Read the model definition and answer for the solid it produces. Units are mm, in the model's axes. Face numbers are marked on the shaded views. Give positions to 0.01 mm unless a question says otherwise; leave off trailing zeros. Order: outer loops, then holes, each group sorted by start corner. A loop starts at its lowest first (then second) coordinate and runs counter-clockwise, first axis right, second up.
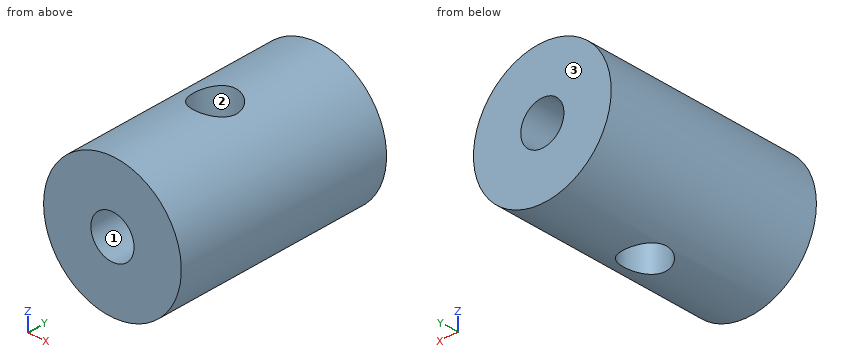
Autodesk Inventor part; units mm, degrees
ref_plane "Work Plane1" through (0, 0, 7.9375) normal (0, 0, 1) x (1, 0, 0)
ref_plane "YZ Plane" through (0, 0, 0) normal (1, 0, 0) x (0, 1, 0)
ref_plane "XZ Plane" through (0, 0, 0) normal (0, 1, 0) x (-1, 0, 0)
sketch "Sketch1" plane through (0, 0, 0) normal (0, 1, 0) x (-1, 0, 0)
  circle A0 centre (0, 0) radius 7.9375
  dimension "d0" = 15.875
extrude "Extrusion1" add sketch "Sketch1" along normal blind 25.4
sketch "Sketch2" plane through (0, 25.4, 0) normal (0, 1, 0) x (1, 0, 0)
  point P0 (0, 0)
  point P1 (0, 0)
hole "Hole1" at (0, 25.4, 0) direction (0, -1, 0) diameter 4.9784 end through all
ref_plane "Work Plane1" through (0, 0, 7.9375) normal (0, 0, 1) x (1, 0, 0)
sketch "Sketch4" plane through (0, 0, 7.9375) normal (0, 0, 1) x (1, 0, 0)
  point P0 (0, 0)
  point P1 (0, 12.7)
  dimension "d11" = 12.7
hole "Hole2" at (0, 12.7, 7.9375) direction (0, 0, -1) diameter 4.9784 end through all
equation "\"d0\" = SlidingTensionerRoundDiameter"
equation "\"d1\" = ShapeWidth"
equation "\"d4\" = ShapeWidth"
equation "\"d13\" = SlidingTensionerRoundDiameter"
equation "\"DrivebaseLength\" = 762"
equation "\"DrivebaseWidth\" = 660.4"
equation "\"ShapeHeight\" = 76.2"
equation "\"ShapeWidth\" = 25.4"
equation "\"ShapeThickness\" = 3.175"
equation "\"WheelDiameter\" = 152.4"
equation "\"WheelRadius\" = 76.2"
equation "\"WheelClearancetoFrame\" = 25.4"
equation "\"SlotLength\" = 88.9"
equation "\"SlotWidth\" = 15.9512"
equation "\"CenterAxleDrop\" = 3.175"
equation "\"CenterAxleXPosition\" = 381"
equation "\"CenterAxleYPosition\" = 25.4"
equation "\"Crossmember1Position\" = 203.2"
equation "\"Crossmember2Position\" = 203.2"
equation "\"CenterlineDrivebaseLength\" = 736.6"
equation "\"CenterlineDrivebaseWidth\" = 635"
equation "\"WheelDistanceFromEdge\" = 101.6"
equation "\"TensionAssemblyJointTravelLengthStart\" = -15.875"
equation "\"SlidingTensionerRoundClearance\" = 0.0762"
equation "\"CenterPointToTensionerRound\" = 28.575"
equation "\"SlidingTensionerRoundDiameter\" = 15.875"
equation "\"TensionAssemblyJointTravelLengthEnd\" = 15.875"
properties part number "200289" material "Steel, Carbon"
1) The part is cut by section D-D on y = 4.5. Determine the outline of the cut face in (x, z) (1 decimal), and give its area (3 significant figures).
Final values:
outline: circle Ø15.9 at (0, 0); hole circle Ø5 at (0, 0)
area: 178 mm2
2) The part is cut by section A-A on x = 0. Determine the outline of the cut face in (y, z).
Final values:
outline: (0, -7.94) - (10.21, -7.94) - (10.21, -2.49) - (0, -2.49) - close; (0, 2.49) - (10.21, 2.49) - (10.21, 7.94) - (0, 7.94) - close; (15.19, -7.94) - (25.4, -7.94) - (25.4, -2.49) - (15.19, -2.49) - close; (15.19, 2.49) - (25.4, 2.49) - (25.4, 7.94) - (15.19, 7.94) - close
3) For a pull along Y with two mould halves and no side action, classify the marked faces 1, 2 and 3 as released by +Y, released by -Y, zero draft, split by the parting line, or undercut.
Final values:
face 1: zero draft
face 2: undercut
face 3: released by +Y
4) The part is cut by section C-C on z = -4.5. Determine the outline of the cut face in (x, y).
Final values:
outline: (-6.54, 0) - (6.54, 0) - (6.54, 25.4) - (-6.54, 25.4) - close; hole circle Ø4.98 at (0, 12.7)
5) Given pin 1 (5 mm diameter, centred on x = -6, y = 11, fed in from +Z); pin 2 (4 mm diameter, centred on x = 0, z = 0, fed in from +Y); pin 3 (2 mm diameter, centred on x = -2.5, y = 17, fed in from +Z); pin 4 (1 mm diameter, centred on x = 5.5, y = 20.5, fed in from -Z), each flat-ended and moving along its own axis, determine where each tip first touches the part or whether it passes through.
Final values:
pin 1: stops at z = 7.12
pin 2: passes through
pin 3: stops at z = 7.79
pin 4: stops at z = -6.16
6) Consider L1, parallel to Y at x = 0, z = -4.75; L2, parallel to Z at x = 0, y = 3.5; L3, parallel to X at y = 15.75, z = -1. Determine where each line is inside the solid, lowest interval first.
Final values:
L1: y = 0 to 10.21, 15.19 to 25.4
L2: z = -7.94 to -2.49, 2.49 to 7.94
L3: x = -7.87 to -2.28, 2.28 to 7.87
